```python
from build123d import *

# Parameters (mm, degrees)
SKETCH1_W           = 20
SKETCH1_H           = 3.8
BOSS_EXTRUDE1_DEPTH = 20
SKETCH2_W           = 3.8
SKETCH2_H           = 20
BOSS_EXTRUDE2_DEPTH = 20
SKETCH3_R           = 5
CUT_EXTRUDE1_DEPTH  = 30
FILLET1_R           = 3


with BuildPart() as part:
    # Sketch1 → Boss-Extrude1 (new body)
    with BuildSketch(Plane.XY):
        with Locations((10, -1.9)):
            Rectangle(SKETCH1_W, SKETCH1_H)
    extrude(amount=BOSS_EXTRUDE1_DEPTH)

    # Sketch2 → Boss-Extrude2 (add)
    with BuildSketch(Plane(origin=(0, 0, 0), x_dir=(1, 0, 0), z_dir=(0, 1, 0))):
        with Locations((18.1, -10)):
            Rectangle(SKETCH2_W, SKETCH2_H)
    extrude(amount=BOSS_EXTRUDE2_DEPTH)

    # Sketch3 → Cut-Extrude1 (cut)
    with BuildSketch(Plane(origin=(0, 0, 0), x_dir=(1, 0, 0), z_dir=(0, 1, 0))):
        with Locations(Location((8.1, -10, 0), (0, 0, 270))):
            Circle(SKETCH3_R)
    extrude(amount=-CUT_EXTRUDE1_DEPTH, mode=Mode.SUBTRACT)

    # Fillet1
    fillet1_edges = [part.edges().sort_by_distance(p)[0] for p in [
        (16.2, 0, 10),
    ]]
    fillet(fillet1_edges, radius=FILLET1_R)


solid = part.part
```
Model file for the job. Use its own axes, mm. A direction names the side the tool comes from. Coordinates: 2 decimals unless noted, no trailing zeros. Order: outer loops, then holes, each group sorted by start corner. A loop starts at its lowest first (then second) coordinate and runs counter-clockwise, first axis right, second up. Notation, with made-up numbers: (-28, -31) -> (-10, -31) arc R25 ccw to (-10, -7) -> close; hole circle Ø2 at (-20, 70.25). An arc over 180 degrees is marked (long way). Answer as a JSON object with one key per item and string values. Group by question number.
1) Drill centre lines: L1, parallel to X at y = -1.7, z = 10; L2, parallel to X at y = 14.5, z = 6.75; L3, parallel to Y at x = 6.5, z = 17.75. Where is each one in solid material? Low to high.
2) Cut at A-A, the plane z = 10. Write the cut outline in (x, y).
3) Flat gauge pins, fed straight in: pin 1 (12 mm diameter, centred on y = 7, z = 16, fed in from -X); pin 2 (1 mm diameter, centred on y = 15.5, z = 13.5, fed in from -X). Where does each tip first touch, or does it go through?
4) Cut at B-B, the plane x = 8.1. Write the cut outline in (y, z).
5) Pull direction Z, two halves, no side cores. Call faces 1 (the face through (14, -3.8, 10)), 2 (the face through (9.6, -1.87, 14.77)), 3 (the face through (17, 5, 0)): +Z half, -Z half, draft (parallel to the pull), parting line (faces both ways), or undercut.
6) Which spindle directions (+Z, -Z, +X, -X, +Y, -Y) get a long thin tool onto all of the face, cutting with end or side? Do faces 4 (the face through (16.2, 11, 10)), 5 (the face through (17, 5, 20)). Say none if no direction does.
7) Cut at D-D, the plane z = 1.5. Write the cut outline in (x, y), then the cut area to 3 significant figures.
8) Cut at C-C, the plane y = -1.25. Write the cut outline in (x, z).
Check values:
{
 "1": {"L1": "x = 0 to 3.1, 13.1 to 20", "L2": "x = 16.2 to 20", "L3": "y = -3.8 to 0"},
 "2": {"outline": "(0, -3.8) -> (3.1, -3.8) -> (3.1, 0) -> (0, 0) -> close; (13.1, -3.8) -> (20, -3.8) -> (20, 20) -> (16.2, 20) -> (16.2, 3) arc R3 cw to (13.2, 0) -> (13.1, 0) -> close"},
 "3": {"pin 1": "stops at x = 15.44", "pin 2": "stops at x = 16.2"},
 "4": {"outline": "(-3.8, 0) -> (0, 0) -> (0, 5) -> (-3.8, 5) -> close; (-3.8, 15) -> (0, 15) -> (0, 20) -> (-3.8, 20) -> close"},
 "5": {"face 1": "draft", "face 2": "undercut", "face 3": "-Z half"},
 "6": {"face 4": "+Z, -Z, -X, +Y", "face 5": "+Z, +X, -X, +Y, -Y"},
 "7": {"outline": "(0, -3.8) -> (20, -3.8) -> (20, 20) -> (16.2, 20) -> (16.2, 3) arc R3 cw to (13.2, 0) -> (0, 0) -> close", "area": "154 mm²"},
 "8": {"outline": "(0, 0) -> (20, 0) -> (20, 20) -> (0, 20) -> close; hole circle Ø10 at (8.1, 10)"}
}
